Here's how the part is built. I have some questions about the finished solid (model axes, mm). A direction names the side the tool comes from. Give positions to 0.01 mm unless a question says otherwise; leave off trailing zeros. Write each loop counter-clockwise with the first axis right and the second up, starting at its lowest first coordinate (ties: lowest second). Pieces come first, ordered by that corner, then holes. Notation, with made-up numbers: (-10.75, 50.5) -> (10.25, 50.5) arc R23 cw to (10.25, 89.5) -> close; hole circle Ø11 at (72, 29.25). An arc over 180 degrees is marked (long way). Use one line per item in the form item = value.
```python
from build123d import *

# Parameters (mm, degrees)
SKETCH_1_R          = 2
EXTRUDE_1_DEPTH     = 4
SKETCH_3_W          = 126
SKETCH_3_H          = 2.7
CUT_EXTRUDE_1_DEPTH = 10
SKETCH_4_R          = 4.5
SKETCH_4_R_2        = 2
CUT_EXTRUDE_2_DEPTH = 10


with BuildPart() as part:
    # 草图1 → 凸台-拉伸1 (new body)
    with BuildSketch(Plane.XY):
        Polygon((145, 46.5), (149, 46.5), (149, 45.15), (151.6, 45.15), (151.6, 46.5), (153.6, 46.5), (153.6, 49.5), (151.6, 49.5), (151.6, 50.85), (149, 50.85), (149, 49.5), (145, 49.5), (145, 59), (141, 59), (141, 67), (145, 67), (145, 76.5), (149, 76.5), (149, 75.15), (151.6, 75.15), (151.6, 76.5), (153.6, 76.5), (153.6, 79.5), (151.6, 79.5), (151.6, 80.85), (149, 80.85), (149, 79.5), (145, 79.5), (145, 89), (141, 89), (141, 97), (145, 97), (145, 106.5), (149, 106.5), (149, 105.15), (151.6, 105.15), (151.6, 106.5), (153.6, 106.5), (153.6, 109.5), (151.6, 109.5), (151.6, 110.85), (149, 110.85), (149, 109.5), (145, 109.5), (145, 123), (271, 123), (271, 109.5), (267, 109.5), (267, 110.85), (264.4, 110.85), (264.4, 109.5), (262.4, 109.5), (262.4, 106.5), (264.4, 106.5), (264.4, 105.15), (267, 105.15), (267, 106.5), (271, 106.5), (271, 97), (275, 97), (275, 89), (271, 89), (271, 79.5), (267, 79.5), (267, 80.85), (264.4, 80.85), (264.4, 79.5), (262.4, 79.5), (262.4, 76.5), (264.4, 76.5), (264.4, 75.15), (267, 75.15), (267, 76.5), (271, 76.5), (271, 67), (275, 67), (275, 59), (271, 59), (271, 49.5), (267, 49.5), (267, 50.85), (264.4, 50.85), (264.4, 49.5), (262.4, 49.5), (262.4, 46.5), (264.4, 46.5), (264.4, 45.15), (267, 45.15), (267, 46.5), (271, 46.5), (271, 37), (275, 37), (275, 29), (271, 29), (271, 19.5), (267, 19.5), (267, 20.85), (264.4, 20.85), (264.4, 19.5), (262.4, 19.5), (262.4, 16.5), (264.4, 16.5), (264.4, 15.15), (267, 15.15), (267, 16.5), (271, 16.5), (271, 7), (275, 7), (275, -1), (271, -1), (271, -10.5), (267, -10.5), (267, -9.15), (264.4, -9.15), (264.4, -10.5), (262.4, -10.5), (262.4, -13.5), (264.4, -13.5), (264.4, -14.85), (267, -14.85), (267, -13.5), (271, -13.5), (271, -27), (271, -34), (145, -34), (145, -27), (145, -13.5), (149, -13.5), (149, -14.85), (151.6, -14.85), (151.6, -13.5), (153.6, -13.5), (153.6, -10.5), (151.6, -10.5), (151.6, -9.15), (149, -9.15), (149, -10.5), (145, -10.5), (145, -1), (141, -1), (141, 7), (145, 7), (145, 16.5), (149, 16.5), (149, 15.15), (151.6, 15.15), (151.6, 16.5), (153.6, 16.5), (153.6, 19.5), (151.6, 19.5), (151.6, 20.85), (149, 20.85), (149, 19.5), (145, 19.5), (145, 29), (141, 29), (141, 37), (145, 37), align=None)
        with Locations((188, 8)):
            Circle(SKETCH_1_R, mode=Mode.SUBTRACT)
        with Locations((228, 8)):
            Circle(SKETCH_1_R, mode=Mode.SUBTRACT)
        with Locations((228, 88)):
            Circle(SKETCH_1_R, mode=Mode.SUBTRACT)
        with Locations((188, 88)):
            Circle(SKETCH_1_R, mode=Mode.SUBTRACT)
    extrude(amount=EXTRUDE_1_DEPTH)

    # 草图3 → 切除-拉伸1 (cut)
    with BuildSketch(Plane.XY.offset(4)):
        with Locations((208, 121.65)):
            Rectangle(SKETCH_3_W, SKETCH_3_H)
    extrude(amount=-CUT_EXTRUDE_1_DEPTH, mode=Mode.SUBTRACT)

    # 草图4 → 切除-拉伸2 (cut)
    with BuildSketch(Plane.XY.offset(4)):
        with Locations((208, 8)):
            Circle(SKETCH_4_R)
        with Locations((228, 48)):
            Circle(SKETCH_4_R_2)
        with Locations((188, 48)):
            Circle(SKETCH_4_R_2)
        with Locations((208, 48)):
            Circle(SKETCH_4_R)
    extrude(amount=-CUT_EXTRUDE_2_DEPTH, mode=Mode.SUBTRACT)


solid = part.part
```
Q1. I want a section at D-D, the plane y = 25. Write out the boundary of the cut face in (x, z).
Result set:
outline = (145, 0) -> (271, 0) -> (271, 4) -> (145, 4) -> close
Q2. I want a section at B-B, the plane x = 208. Write out the boundary of the cut face in (y, z).
Result set:
outline = (-34, 0) -> (3.5, 0) -> (3.5, 4) -> (-34, 4) -> close; (12.5, 0) -> (43.5, 0) -> (43.5, 4) -> (12.5, 4) -> close; (52.5, 0) -> (120.3, 0) -> (120.3, 4) -> (52.5, 4) -> close
Q3. Which directions (+Z, -Z, +X, -X, +Y, -Y) give clear straight access to the entire face, cutting with the end or side of a thin tool? Please do faces 1 (the face through (145, 115, 2)), 2 (the face through (143, 89, 2)), 3 (the face through (271, -24, 2)), 4 (the face through (271, 72, 2)), 5 (the face through (212.16, 6.28, 2.03)).
Result set:
face_1 = +Z, -Z, -X, +Y
face_2 = +Z, -Z, -X
face_3 = +Z, -Z, +X, -Y
face_4 = +Z, -Z, +X
face_5 = +Z, -Z
Q4. Will these pins go through, and if not, where does the flat tip stop? pin 1 Ø1.1 at (y, z) = (-14, 2) entering from -X; pin 2 Ø1.5 at (y, z) = (17.5, 1.5) entering from -X; pin 3 Ø1.1 at (y, z) = (106, 1) entering from +X; pin 4 Ø3.5 at (x, y) = (188, 88) entering from -Z.
Result set:
pin_1 = 145
pin_2 = 153.6
pin_3 = 271
pin_4 = through
Q5. I want a section at A-A, the plane x = 228. Write out the boundary of the cut face in (y, z).
Result set:
outline = (-34, 0) -> (6, 0) -> (6, 4) -> (-34, 4) -> close; (10, 0) -> (46, 0) -> (46, 4) -> (10, 4) -> close; (50, 0) -> (86, 0) -> (86, 4) -> (50, 4) -> close; (90, 0) -> (120.3, 0) -> (120.3, 4) -> (90, 4) -> close
Q6. If we mould it in two halves opening along Y, with no side actions, what happens to faces 6 (the face through (145, 102, 2)), 7 (the face through (145, 24, 2)), 8 (the face through (143, -1, 2))? For each: +Y half, -Y half, draft (parallel to the pull), parting line (faces both ways), or undercut.
Result set:
face_6 = draft
face_7 = undercut
face_8 = -Y half
Q7. If I drill on line 1 along Y through (x, z) = (150, 1.65); line 2 along Y through (x, z) = (188, 2.8); line 3 along X through (y, z) = (105.5, 0.3), over which ranges is the centre line in solid material (lowest first)? Write a range as from..to.
Result set:
line_1 = -34..-14.85, -9.15..15.15, 20.85..45.15, 50.85..75.15, 80.85..105.15, 110.85..120.3
line_2 = -34..6, 10..46, 50..86, 90..120.3
line_3 = 145..149, 151.6..264.4, 267..271
Q8. I want a section at C-C, the plane z = 3.3. Count the separate pieces of the cut face and the enclosed holes in it, and give its area (3 significant figures).
Result set:
separate_pieces = 1
enclosed_holes = 8
area = 19,200 mm2
